```python
from build123d import *

# Parameters (mm, degrees)
F1_DEPTH = 3
F2_R     = 4.75
F3_DEPTH = 1
F4_W     = 28
F4_H     = 16
F5_DEPTH = 5
F7_D     = 3.3
F7_DEPTH = 5
F7_TIP   = 0.9914200214


with BuildPart() as f1:
    # F0 (on Top) → F1 (new body)
    with BuildSketch(Plane.XY):
        Polygon((23, 10), (-26, 10), (-26, -10), (26, -10), (26, -1), align=None)
    extrude(amount=-F1_DEPTH)

    # F2 (on face) → F3 (cut)
    with BuildSketch(Plane(origin=(0, 0, -3), x_dir=(1, 0, 0), z_dir=(0, 0, -1))):
        with Locations((19, 3)):
            Circle(F2_R)
        with Locations((6.3, 2.3)):
            Circle(F2_R)
        with Locations((-6.4, 1.7)):
            Circle(F2_R)
        with Locations((-19.1, 1)):
            Circle(F2_R)
    extrude(amount=-F3_DEPTH, mode=Mode.SUBTRACT)

    # F4 (on face) → F5 (join)
    with BuildSketch(Plane.XY):
        with Locations((7, 2)):
            Rectangle(F4_W, F4_H)
    extrude(amount=F5_DEPTH)

    # F7
    with Locations(Plane.XY.offset(5)):
        with Locations((0, 2), (12, 2)):
            Hole(F7_D / 2, depth=F7_DEPTH)
            with Locations((0, 0, -(F7_DEPTH + F7_TIP / 2))):  # 118° drill point
                Cone(0, F7_D / 2, F7_TIP, mode=Mode.SUBTRACT)


solid = f1.part
```
The listing builds one solid part. Answer for the finished solid, in the listing's coordinates (mm). A direction names the side the tool comes from. Round coordinates to 2 decimals unless told otherwise and drop trailing zeros. Loops run counter-clockwise (first coordinate to the right, second up) from the corner with the lowest first, then second, coordinate; pieces in that order, holes last. Notation, with made-up numbers: (75.25, 0.25) -> (107.25, 0.25) arc R22 cw to (107.25, 27.25) -> close; hole circle Ø4 at (48.25, 35.5). An arc over 180 degrees is marked (long way). Use one line per item in the form item = value.
1. A tool of negligible diameter and unlimited length cuts with its end or side. For faces 1 (the flat face through (-7, 2, 2)), 2 (the cylindrical face through (0.215, 3.636, 2.465)), 3 (the cylindrical face through (-22.87, 1.89, -2.51)), 4 (the flat face through (21, 2, 2)), 5 (the flat face through (-26, 0, -1)), from which of +Z, -Z, +X, -X, +Y, -Y can it reach the whole face along a straight path? Write none if from no direction.
Answer key:
face_1 = +Z, -X, +Y, -Y
face_2 = +Z
face_3 = -Z
face_4 = +Z, +X, +Y, -Y
face_5 = +Z, -Z, -X, +Y, -Y
2. Find the intervals of material crossed by probe 1 along X at (y, z) = (2, 2.05); probe 2 along Y at (x, z) = (12, 3.65); probe 3 along Y at (x, z) = (-19.1, -2.45), in increasing order. Write a range as [from, to].
Answer key:
probe_1 = [-7, -1.65], [1.65, 10.35], [13.65, 21]
probe_2 = [-6, 0.35], [3.65, 10]
probe_3 = [-10, -5.75], [3.75, 10]
3. The part is cut by section A-A on z = 1.75. Determine the outline of the cut face in (x, y).
Answer key:
outline = (-7, -6) -> (21, -6) -> (21, 10) -> (-7, 10) -> close; hole circle Ø3.3 at (0, 2); hole circle Ø3.3 at (12, 2)
4. For a pull along Y with two mould halves and no side action, classify faces 6 (the flat face through (-6, -2, -2)), 7 (the flat face through (7, 2, 5)), 8 (the flat face through (7, -6, 2)) as released by +Y, released by -Y, zero draft, split by the parting line, or undercut.
Answer key:
face_6 = undercut
face_7 = zero draft
face_8 = released by -Y
5. The part is cut by section C-C on z = -2.5. Determine the outline of the cut face in (x, y).
Answer key:
outline = (-26, -10) -> (26, -10) -> (26, -1) -> (23, 10) -> (-26, 10) -> close; hole circle Ø9.5 at (-19.1, -1); hole circle Ø9.5 at (-6.4, -1.7); hole circle Ø9.5 at (6.3, -2.3); hole circle Ø9.5 at (19, -3)
6. Flat-ended cylindrical pins translate along their axes: pin 1 Ø8 at (x, y) = (-16.5, -6.5) entering from +Z; pin 2 Ø5 at (x, y) = (17, -2.5) entering from -Z; pin 3 Ø2.5 at (y, z) = (6, 2) entering from +X; pin 4 Ø1 at (y, z) = (-7, 1.5) entering from -X. Find the tip coordinate at first contact, or state that the pin passes through.
Answer key:
pin_1 = 0
pin_2 = -2
pin_3 = 21
pin_4 = through
7. The part is cut by section B-B on x = 6.3. Determine the outline of the cut face in (y, z), and give its area (4 significant figures).
Answer key:
outline = (-10, -3) -> (-7.05, -3) -> (-7.05, -2) -> (2.45, -2) -> (2.45, -3) -> (10, -3) -> (10, 5) -> (-6, 5) -> (-6, 0) -> (-10, 0) -> close
area = 130.5 mm²
8. The part is cut by section D-D on y = -4.5. Determine the outline of the cut face in (x, z).
Answer key:
outline = (-26, -3) -> (-22.31, -3) -> (-22.31, -2) -> (-15.89, -2) -> (-15.89, -3) -> (-10.24, -3) -> (-10.24, -2) -> (-2.56, -2) -> (-2.56, -3) -> (2.09, -3) -> (2.09, -2) -> (10.51, -2) -> (10.51, -3) -> (14.49, -3) -> (14.49, -2) -> (23.51, -2) -> (23.51, -3) -> (26, -3) -> (26, 0) -> (21, 0) -> (21, 5) -> (-7, 5) -> (-7, 0) -> (-26, 0) -> close
